Source: CAD feature listing. Evaluate the final solid. Frame: model axes, mm. Face numbers are marked on the shaded views. Coordinates: 2 decimals unless noted, no trailing zeros. Order: outer loops, then holes, each group sorted by start corner. A loop starts at its lowest first (then second) coordinate and runs counter-clockwise, first axis right, second up.
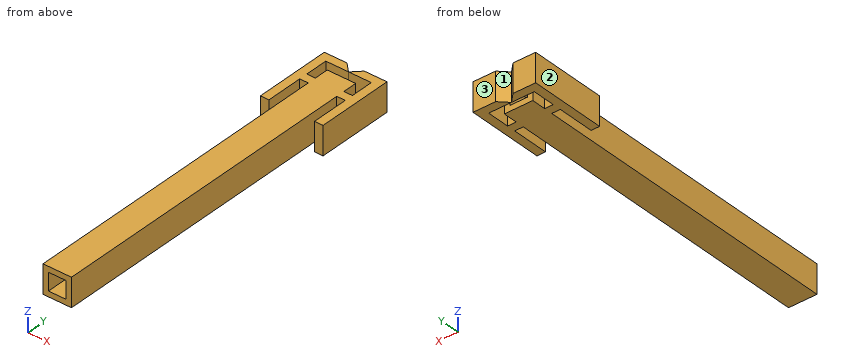
```python
from build123d import *

# Parameters (mm, degrees)
F0_W     = 1.5
F0_H     = 6.5
F1_DEPTH = 5
F3_W     = 3.08
F3_H     = 3.08
F4_DEPTH = 60


with BuildPart() as f1:
    # F0 (on Top) → F1 (new body)
    with BuildSketch(Plane.XY):
        Polygon((-1.25, -30), (1.25, -30), (1.25, 26), (1.25, 27.5), (1.25, 30), (-1.25, 30), align=None)
        Polygon((1.25, 27.5), (1.25, 26), (2.75, 26), (4.25, 26), (4.25, 33), (0.27, 33), (-1.23, 31.5), (2.75, 31.5), (2.75, 27.5), align=None)
        with Locations((3.5, 22.75)):
            Rectangle(F0_W, F0_H)
    extrude(amount=F1_DEPTH)

    # F2: F1 across face


with BuildPart() as f1_1:
    add(f1.part)
    add(f1.part.mirror(Plane(origin=(-1.25, 0, 2.5), x_dir=(0, -1, 0), z_dir=(-1, 0, 0))))

    # F3 (on face) → F4 (cut, through all)
    with BuildSketch(Plane.XZ.offset(30)):
        with Locations((-1.25, 2.5)):
            Rectangle(F3_W, F3_H)
    extrude(amount=-F4_DEPTH, mode=Mode.SUBTRACT)


solid = f1_1.part
```
1. Section query A-A on y = 22.5. Return loops of the section in (x, z).
Findings:
outline: (-6.75, 0) - (-5.25, 0) - (-5.25, 5) - (-6.75, 5) - close; (-3.75, 0) - (1.25, 0) - (1.25, 5) - (-3.75, 5) - close; (2.75, 0) - (4.25, 0) - (4.25, 5) - (2.75, 5) - close; hole (-2.79, 0.96) - (0.29, 0.96) - (0.29, 4.04) - (-2.79, 4.04) - close
2. Section query B-B on x = -2. Return loops of the section in (y, z).
Findings:
outline: (-30, 0) - (30, 0) - (30, 0.96) - (-30, 0.96) - close; (-30, 4.04) - (30, 4.04) - (30, 5) - (-30, 5) - close; (31.5, 0) - (32.23, 0) - (32.23, 5) - (31.5, 5) - close
3. Ray query, line 1 (X direction, y = 23, z = 3.8); line 2 (X direction, y = 21.5, z = 4.4); line 3 (X direction, y = -24, z = 3.6). Return the intervals inside material, ascending.
Findings:
line 1: x = -6.75 to -5.25, -3.75 to -2.79, 0.29 to 1.25, 2.75 to 4.25
line 2: x = -6.75 to -5.25, -3.75 to 1.25, 2.75 to 4.25
line 3: x = -3.75 to -2.79, 0.29 to 1.25
4. Draft query along X for the marked faces 1, 2 and 3. Return one class per face: released by +X, released by -X, zero draft, split by the parting line, or undercut.
Findings:
face 1: undercut
face 2: released by -X
face 3: zero draft
5. Section query D-D on y = -25. Return loops of the section in (x, z).
Findings:
outline: (-3.75, 0) - (1.25, 0) - (1.25, 5) - (-3.75, 5) - close; hole (-2.79, 0.96) - (0.29, 0.96) - (0.29, 4.04) - (-2.79, 4.04) - close
6. Pin query (flat end, axial travel): P1, Ø2.5, axis at y = -0.5, z = 3, coming from the +X side; P2, Ø2.5, axis at y = -9, z = 3, coming from the -X side; P3, Ø1.2, axis at x = -6, z = 2, coming from the -Y side. Return the tip coordinate at first contact, or that it passes through.
Findings:
P1: stops at x = 1.25
P2: stops at x = -3.75
P3: stops at y = 19.5
7. Section query C-C on z = 1.65. Return loops of the section in (x, y), plus the area to 3 significant figures.
Findings:
outline: (-6.75, 19.5) - (-5.25, 19.5) - (-5.25, 26) - (-3.75, 26) - (-3.75, -30) - (-2.79, -30) - (-2.79, 30) - (-3.75, 30) - (-3.75, 27.5) - (-5.25, 27.5) - (-5.25, 31.5) - (-1.27, 31.5) - (-2.77, 33) - (-6.75, 33) - close; (-1.23, 31.5) - (2.75, 31.5) - (2.75, 27.5) - (1.25, 27.5) - (1.25, 30) - (0.29, 30) - (0.29, -30) - (1.25, -30) - (1.25, 26) - (2.75, 26) - (2.75, 19.5) - (4.25, 19.5) - (4.25, 33) - (0.27, 33) - close
area: 170 mm2
